Geometry check sheet. Reference: the model listing, model coordinates, mm. A direction names the side the tool comes from. Give positions to 0.01 mm unless a question says otherwise; leave off trailing zeros. Write each loop counter-clockwise with the first axis right and the second up, starting at its lowest first coordinate (ties: lowest second). Pieces come first, ordered by that corner, then holes.
(1) Thickness scan on line 1 along Z through (x, y) = (102, 18.75); line 2 along Y through (x, z) = (105, 10.45); line 3 along Y through (x, z) = (103.25, 10.9). Record the ranges inside material, lowest first.
(2) Cross-section at A-A (x = 102.31). Record the boundary of the cut face in (y, z).
(3) Tool access check on faces 1 (the cylindrical face through (106.125, 25.411, 9.032)), 2 (the flat face through (102, 24, 11.3)). Record the directions out of +Z, -Z, +X, -X, +Y, -Y that give a thin tool (end or side, any length) a straight path to the whole face; none if there is none.
(4) Cross-section at C-C (z = 8.2). Record the boundary of the cut face in (x, y).
(5) Cross-section at B-B (y = 24.21). Record the boundary of the cut face in (x, z), and give its area (3 significant figures).
(6) Cross-section at D-D (x = 97). Record the boundary of the cut face in (y, z).
(7) Depth check by flat-ended pin: P1, Ø1, axis at x = 97.5, z = 10.5, coming from the +Y side; P2, Ø1, axis at x = 102, z = 9, coming from the +Y side; P3, Ø2, axis at x = 104, z = 7, coming from the -Y side. Enter the tip coordinate at first touch or a pass-through.
```python
from build123d import *

# Parameters (mm, degrees)
BOX117_W          = 10
BOX117_H          = 10
BOX117_DEPTH      = 10
CYLINDER013_R     = 4
CYLINDER013_DEPTH = 5
FILLET001_R       = 1
CYLINDER014_R     = 6.25
CYLINDER014_DEPTH = 1.5


with BuildPart() as cube107:
    # Box117 → Box117 (new body)
    with BuildSketch(Plane(origin=(97.4, 28.4, 0), x_dir=(1, 0, 0), z_dir=(0, 0, 1))):
        with Locations((5, 5)):
            Rectangle(BOX117_W, BOX117_H)
    extrude(amount=BOX117_DEPTH)


with BuildPart() as obj1:
    # Cylinder013 → Cylinder013 (new body)
    with BuildSketch(Plane(origin=(120.31, 24.21, 6.3), x_dir=(1, 0, 0), z_dir=(0, 0, 1))):
        Circle(CYLINDER013_R)
    extrude(amount=CYLINDER013_DEPTH)

    # Fillet001
    fillet001_edges = [obj1.edges().sort_by_distance(p)[0] for p in [
        (116.31, 24.21, 11.3),
    ]]
    fillet(fillet001_edges, radius=FILLET001_R)


with BuildPart() as cut073:
    # Cylinder014 → Cylinder014 (new body)
    with BuildSketch(Plane(origin=(120.31, 24.21, 6.3), x_dir=(1, 0, 0), z_dir=(0, 0, 1))):
        Circle(CYLINDER014_R)
    extrude(amount=CYLINDER014_DEPTH)

    # Fusion013: union obj1
    add(obj1.part)


with BuildPart() as cut073_1:
    # Fusion013 placement: moved
    add(cut073.part.moved(Location((-18, 0, 0))))

    # Cut073: cut Cube107
    add(cube107.part, mode=Mode.SUBTRACT)


solid = cut073_1.part
```
Reply:
1. line 1: z = 6.3 to 7.8
1. line 2: y = 21.26 to 27.16
1. line 3: y = 20.53 to 27.89
2. outline: (17.96, 6.3) - (28.4, 6.3) - (28.4, 7.8) - (28.21, 7.8) - (28.21, 10.3) arc R1 ccw to (27.21, 11.3) - (21.21, 11.3) arc R1 ccw to (20.21, 10.3) - (20.21, 7.8) - (17.96, 7.8) - close
3. face 1: +Z
3. face 2: +Z, +X, -X, +Y, -Y
4. outline: circle Ø8 at (102.31, 24.21)
5. outline: (96.06, 6.3) - (108.56, 6.3) - (108.56, 7.8) - (106.31, 7.8) - (106.31, 10.3) arc R1 ccw to (105.31, 11.3) - (99.31, 11.3) arc R1 ccw to (98.31, 10.3) - (98.31, 7.8) - (96.06, 7.8) - close
5. area: 46.3 mm2
6. outline: (20.91, 6.3) - (27.51, 6.3) - (27.51, 7.8) - (20.91, 7.8) - close
7. P1: passes through
7. P2: stops at y = 28.21
7. P3: stops at y = 18
